Autodesk Inventor part; units mm, degrees
ref_plane "Belt Plane" through (0, 31, 8) normal (0, 0, 1) x (1, 0, 0)
ref_plane "YZ Plane" through (0, 0, 0) normal (1, 0, 0) x (0, 1, 0)
ref_plane "XZ Plane" through (0, 0, 0) normal (0, 1, 0) x (-1, 0, 0)
sketch "Main Sketch" plane through (0, 0, 0) normal (1, 0, 0) x (0, 1, 0)
  line L0 (0, 16) -> (42, 16)
  line L1 (42, 16) -> (42, 12.8615)
  line L2 (42, 12.8615) -> (31, 9.4984)
  line L3 (31, 9.4984) -> (31, 6.5016)
  line L4 (31, 6.5016) -> (42, 3.1385)
  line L5 (42, 3.1385) -> (42, 0)
  line L6 (42, 0) -> (0, 0)
  line L7 (40, 12.25) -> (40, 3.75) construction
  line L8 (31, 8) -> (40, 8) construction
  line L9 (42, 12.8615) -> (42, 3.1385)
  line L10 (0, -4) -> (0, 24)
  line L11 (0, 0) -> (0, 16)
  dimension "d0" = 8.5
  dimension "d1" = 34
  dimension "d2" = 2
  dimension "d6" = 16
  dimension "d21" = 80
  dimension "d25" = 11
  dimension "d27" = 8
ref_plane "Belt Plane" through (0, 31, 8) normal (0, 0, 1) x (1, 0, 0)
revolve "Body" add sketch "Main Sketch" angle 360 about axis through (0, 0, -10) along (0, 0, 1)
revolve "Groove" cut sketch "Main Sketch" angle 360 about axis through (0, 0, -10) along (0, 0, 1) contours L9 L4 L3 L2
fillet "Fillet External" [suppressed]
fillet "Fillet Internal" [suppressed]
pattern_of_one "Groove Pattern"
equation "\"d0\" = da_Bw"
equation "\"d1\" = da_Alfa"
equation "\"d2\" = da_c"
equation "\"d21\" = da_Dw"
equation "\"d25\" = da_Hd"
equation "\"d27\" = da_Se"
equation "\"da_r1\" = 0"
equation "\"da_r2\" = 0"
equation "\"d18\" = da_Sg"
equation "\"d5\" = da_Se"
equation "\"da_Bw\" = 8.5"
equation "\"da_Alfa\" = 34deg"
equation "\"da_c\" = 2"
equation "\"da_Dw\" = 80"
equation "\"da_Hd\" = 11"
equation "\"da_Se\" = 8"
equation "\"da_Sg\" = 12"
properties part number "Grooved Pulley2" material "Steel"
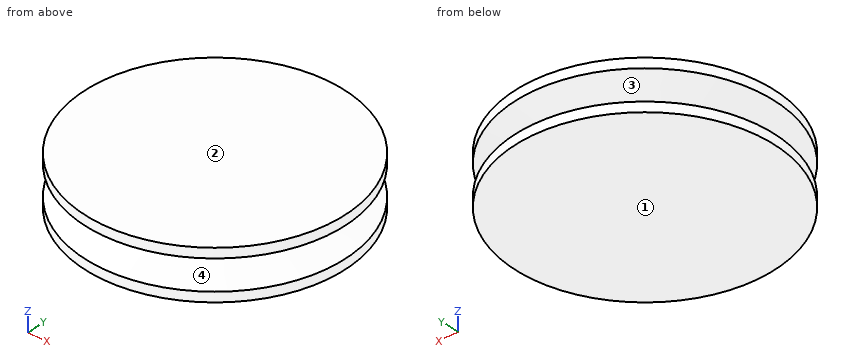
Input: part model. Units: mm. Frame: model coordinates. Face numbers are marked on the shaded views. Give positions to 0.01 mm unless a question says otherwise; leave off trailing zeros. Write each loop counter-clockwise with the first axis right and the second up, starting at its lowest first coordinate (ties: lowest second). Pieces come first, ordered by that corner, then holes.
Q1. Material intervals for probe 1 along Z at (x, y) = (29, -14); probe 2 along Z at (x, y) = (17, -37); probe 3 along X at (y, z) = (-16, 1), sorted ascending.
Q2. First-contact query: P1, Ø5, axis at y = 10.5, z = 4.5, coming from the -X side; P2, Ø6, axis at y = 17.5, z = 4, coming from the -X side. Flat tips, straight axial feed; report the tip coordinate or a pass-through.
Q3. Pull-direction query (Z, two-part tool) for the marked faces 1, 2, 3 and 4; classes: pulls with the +Z half, pulls with the -Z half, needs draft (parallel to the pull), parting line crosses it, or undercut.
Q4. Section D-D, the plane z = 10.5. Output: boundary loops of the cut face in (x, y), plus the area to 3 significant figures.
Q5. Section C-C, the plane z = 15. Output: boundary loops of the cut face in (x, y), plus the area to 3 significant figures.
Q6. Section A-A, the plane y = 0. Output: boundary loops of the cut face in (x, z).
Filled in:
1. probe 1: z = 0 to 6.13, 9.87 to 16
1. probe 2: z = 0 to 3.53, 12.47 to 16
1. probe 3: x = -38.83 to 38.83
2. P1: stops at x = -41.15
2. P2: stops at x = -39.37
3. face 1: pulls with the -Z half
3. face 2: pulls with the +Z half
3. face 3: undercut
3. face 4: undercut
4. outline: circle Ø68.55 at (0, 0)
4. area: 3,690 mm2
5. outline: circle Ø84 at (0, 0)
5. area: 5,540 mm2
6. outline: (-42, 0) - (42, 0) - (42, 3.14) - (31, 6.5) - (31, 9.5) - (42, 12.86) - (42, 16) - (-42, 16) - (-42, 12.86) - (-31, 9.5) - (-31, 6.5) - (-42, 3.14) - close
